Geometry check sheet. Reference: the model listing, model coordinates, mm. A direction names the side the tool comes from. Give positions to 0.01 mm unless a question says otherwise; leave off trailing zeros. Loops run counter-clockwise (first coordinate to the right, second up) from the corner with the lowest first, then second, coordinate; pieces in that order, holes last. Notation, with made-up numbers: (34, -14.5) -> (80, -14.5) arc R11 ccw to (80, -4.5) -> close; hole circle Ø2 at (-39.5, 0.25). An arc over 180 degrees is marked (long way). Write item = value, one per line.
Autodesk Inventor part; units mm, degrees
ref_plane "YZ Plane" through (0, 0, 0) normal (1, 0, 0) x (0, 1, 0)
ref_plane "XZ Plane" through (0, 0, 0) normal (0, 1, 0) x (-1, 0, 0)
ref_plane "XY Plane" through (0, 0, 0) normal (0, 0, 1) x (1, 0, 0)
sketch "Sketch1" plane through (0, 0, 0) normal (0, 1, 0) x (-1, 0, 0)
  line L0 (-22, -14.1429) -> (-22, 15.8571)
  line L1 (-20.3963, 17.8571) -> (20.3963, 17.8571)
  line L2 (22, 15.8571) -> (22, -14.1429)
  arc A0 (-22, -14.1429) -> (22, -14.1429) centre (0, -14.1429) ccw
  line L3 (20.3963, 17.8571) -> (30.3963, 17.8571)
  line L4 (30.3963, 17.8571) -> (30.3963, 15.8571)
  line L5 (30.3963, 15.8571) -> (22, 15.8571)
  line L6 (-20.3963, 17.8571) -> (-30.3963, 17.8571)
  line L7 (-30.3963, 17.8571) -> (-30.3963, 15.8571)
  line L8 (-30.3963, 15.8571) -> (-22, 15.8571)
  point P0 (0, 0)
  point P1 (0, 17.8571)
  point P2 (22, 0)
  dimension "d1" = 2
  dimension "d2" = 2
  dimension "d3" = 10
  dimension "d4" = 10
  dimension "d5" = 30
  dimension "d6" = 22
extrude "Extrusion1" add sketch "Sketch1" along normal mid plane 30
sketch "Sketch2" plane through (0, 15, 0) normal (0, 1, 0) x (1, 0, 0)
  line L0 (-15, 14.8429) -> (-10, 14.8429)
  line L1 (-10, 14.8429) -> (-10, 19.8429)
  line L2 (-10, 19.8429) -> (10, 19.8429)
  line L3 (10, 19.8429) -> (10, 14.8429)
  line L4 (10, 14.8429) -> (15, 14.8429)
  line L5 (15, 14.8429) -> (15, 17.1429)
  line L6 (15, 17.1429) -> (12.3, 17.1429)
  line L7 (12.3, 17.1429) -> (12.3, 22.1429)
  line L8 (12.3, 22.1429) -> (-12.3, 22.1429)
  line L9 (-12.3, 22.1429) -> (-12.3, 17.1429)
  line L10 (-12.3, 17.1429) -> (-15, 17.1429)
  line L11 (-15, 17.1429) -> (-15, 14.8429)
  arc A0 (22, 14.1429) -> (-22, 14.1429) centre (0, 14.1429) ccw
  point P0 (0, 0)
  point P1 (0, 22.1429)
  point P2 (0, 19.8429)
  point P3 (0, 36.1429)
  point P4 (15, 15.9929)
  point P5 (-15, 15.9929)
  point P6 (10, 17.3429)
  point P7 (-10, 17.3429)
  point P8 (-12.5, 14.8429)
  point P9 (-13.65, 17.1429)
  dimension "d9" = 14
  dimension "d11" = 2.3
  dimension "d13" = 24.6
  dimension "d14" = 20
  dimension "d15" = 5
  dimension "d17" = 5
  dimension "d27" = 2.3
extrude "Extrusion2" cut sketch "Sketch2" against normal blind 25
sketch "Sketch3" plane through (30.3963, 15, 15.8571) normal (0, 0, -1) x (-1, 0, 0)
  line L0 (0, -30) -> (0, 0)
  line L1 (0, 0) -> (8.3963, 0)
  point P0 (30.3963, -15)
  point P1 (4.1982, -15)
  point P2 (0, -15)
  point P3 (4.1982, 0)
hole "Hole1" at (26.1982, 0, 15.8571) direction (0, 0, 1) diameter 3 depth 2
mirror "Mirror1" about plane through (0, 0, 0) normal (1, 0, 0) of "Hole1"
properties part number "Part_B7"
Item 1: Section check D-D, the plane x = 0. Record the cut outline in (y, z), plus the area to 3 significant figures.
Answer:
outline = (-15, -36.14) -> (15, -36.14) -> (15, -22.14) -> (-10, -22.14) -> (-10, -19.84) -> (15, -19.84) -> (15, 17.86) -> (-15, 17.86) -> close
area = 1,560 mm^2
Item 2: Section check A-A, the plane y = 0. Record the cut outline in (x, z).
Answer:
outline = (-30.4, 15.86) -> (-27.7, 15.86) -> (-27.7, 17.86) -> (-30.4, 17.86) -> close; (-24.7, 15.86) -> (-22, 15.86) -> (-22, -14.14) arc R22 ccw to (22, -14.14) -> (22, 15.86) -> (24.7, 15.86) -> (24.7, 17.86) -> (-24.7, 17.86) -> close; (27.7, 15.86) -> (30.4, 15.86) -> (30.4, 17.86) -> (27.7, 17.86) -> close; hole (-15, -17.14) -> (-12.3, -17.14) -> (-12.3, -22.14) -> (12.3, -22.14) -> (12.3, -17.14) -> (15, -17.14) -> (15, -14.84) -> (10, -14.84) -> (10, -19.84) -> (-10, -19.84) -> (-10, -14.84) -> (-15, -14.84) -> close
Item 3: Gauge pin test, flat ends, axial feed: pin 1 (5.5 mm diameter, centred on y = 8.5, z = -19, fed in from +X); pin 2 (1.5 mm diameter, centred on x = 11.5, y = 3, fed in from -Z); pin 3 (3.5 mm diameter, centred on x = 26.2, y = 0, fed in from -Z). Record the tip position at first contact, or that the pin passes through.
Answer:
pin_1 = 21.9
pin_2 = -33.34
pin_3 = 15.86
Item 4: Section check C-C, the plane z = -19. Record the cut outline in (x, y), plus the area to 3 significant figures.
Answer:
outline = (-21.46, -15) -> (21.46, -15) -> (21.46, 15) -> (12.3, 15) -> (12.3, -10) -> (10, -10) -> (10, 15) -> (-10, 15) -> (-10, -10) -> (-12.3, -10) -> (-12.3, 15) -> (-21.46, 15) -> close
area = 1,170 mm^2
Item 5: Draft check along X on faces 1 (the flat face through (-28, 0, 15.857)), 2 (the cylindrical face through (-27.685, -0.195, 16.871)), 3 (the flat face through (-22, 0, 1)). Enter one of: +X half, -X half, draft (parallel to the pull), parting line (faces both ways), or undercut.
Answer:
face_1 = draft
face_2 = undercut
face_3 = -X half
Item 6: Thickness scan on L1, parallel to X at y = 0, z = 16.85; L2, parallel to X at y = 14.25, z = -15.5; L3, parallel to X at y = -4.75, z = 7.5. Record the ranges inside material, lowest first. Write a range as [from, to].
Answer:
L1 = [-30.4, -27.7], [-24.7, 24.7], [27.7, 30.4]
L2 = [-21.96, -15], [-10, 10], [15, 21.96]
L3 = [-22, 22]
Item 7: Tool access check on faces 4 (the flat face through (22, 0, 1)), 5 (the flat face through (0, -15, -9)), 6 (the flat face through (-10, 3, -17)). Record the directions out of +Z, -Z, +X, -X, +Y, -Y that give a thin tool (end or side, any length) a straight path to the whole face; none if there is none.
Answer:
face_4 = -Z, +X, +Y, -Y
face_5 = +Z, -Z, +X, -X, -Y
face_6 = +Y
Item 8: Section check B-B, the plane y = -6.5. Record the cut outline in (x, z).
Answer:
outline = (-30.4, 15.86) -> (-22, 15.86) -> (-22, -14.14) arc R22 ccw to (22, -14.14) -> (22, 15.86) -> (30.4, 15.86) -> (30.4, 17.86) -> (-30.4, 17.86) -> close; hole (-15, -17.14) -> (-12.3, -17.14) -> (-12.3, -22.14) -> (12.3, -22.14) -> (12.3, -17.14) -> (15, -17.14) -> (15, -14.84) -> (10, -14.84) -> (10, -19.84) -> (-10, -19.84) -> (-10, -14.84) -> (-15, -14.84) -> close
